```python
from build123d import *

# Parameters (mm, degrees)
BOSS_EXTRUDE1_DEPTH = 30
SKETCH16_W          = 33.4
SKETCH16_H          = 12.9
CUT_EXTRUDE10_DEPTH = 4.5
SKETCH17_W          = 23.45208563
SKETCH17_H          = 12.9
CUT_EXTRUDE11_DEPTH = 192.865838543
CUT_EXTRUDE13_DEPTH = 6.45
SKETCH19_R          = 20
CUT_EXTRUDE14_DEPTH = 8.8
SKETCH21_W          = 33.4
SKETCH21_H          = 12.9
CUT_EXTRUDE15_DEPTH = 191.957455995
SKETCH23_R          = 1.1
CUT_EXTRUDE16_DEPTH = 192.865838543


with BuildPart() as part:
    # Sketch1 → Boss-Extrude1 (new body)
    with BuildSketch(Plane.XY):
        with BuildLine():
            ThreePointArc((187.5, 0), (167.823244805, 26.363741023), (136.951138857, 15))
            Line((136.951138857, 15), (160, 15))
            Line((160, 15), (160, -15))
            Line((160, -15), (136.951138857, -15))
            ThreePointArc((136.951138857, -15), (167.823244805, -26.363741023), (187.5, 0))
        make_face()
        with BuildLine():
            Line((160, 15), (136.951138857, 15))
            ThreePointArc((136.951138857, 15), (132.5, 0), (136.951138857, -15))
            Line((136.951138857, -15), (160, -15))
            Line((160, -15), (160, 15))
        make_face()
        with BuildLine():
            Line((136.951138857, 15), (23.048861143, 15))
            ThreePointArc((23.048861143, 15), (26.363741023, 7.823244805), (27.5, 0))
            ThreePointArc((27.5, 0), (26.363741023, -7.823244805), (23.048861143, -15))
            Line((23.048861143, -15), (136.951138857, -15))
            ThreePointArc((136.951138857, -15), (132.5, 0), (136.951138857, 15))
        make_face()
        with BuildLine():
            ThreePointArc((13.228756555, -15), (-20, 0), (13.228756555, 15))
            Line((13.228756555, 15), (23.048861143, 15))
            ThreePointArc((23.048861143, 15), (-27.5, 0), (23.048861143, -15))
            Line((23.048861143, -15), (13.228756555, -15))
        make_face()
        with BuildLine():
            Line((23.048861143, 15), (13.228756555, 15))
            ThreePointArc((13.228756555, 15), (18.228756555, 8.228756555), (20, 0))
            ThreePointArc((20, 0), (18.228756555, -8.228756555), (13.228756555, -15))
            Line((13.228756555, -15), (23.048861143, -15))
            ThreePointArc((23.048861143, -15), (26.363741023, -7.823244805), (27.5, 0))
            ThreePointArc((27.5, 0), (26.363741023, 7.823244805), (23.048861143, 15))
        make_face()
        with BuildLine():
            Line((0, -15), (0, 15))
            Line((0, 15), (13.228756555, 15))
            ThreePointArc((13.228756555, 15), (-20, 0), (13.228756555, -15))
            Line((13.228756555, -15), (0, -15))
        make_face()
        with BuildLine():
            Line((13.228756555, 15), (0, 15))
            Line((0, 15), (0, -15))
            Line((0, -15), (13.228756555, -15))
            ThreePointArc((13.228756555, -15), (18.228756555, -8.228756555), (20, 0))
            ThreePointArc((20, 0), (18.228756555, 8.228756555), (13.228756555, 15))
        make_face()
    extrude(amount=BOSS_EXTRUDE1_DEPTH)

    # Sketch16 → Cut-Extrude10 (cut)
    with BuildSketch(Plane(origin=(0, 0, 0), x_dir=(-1, 0, 0), z_dir=(0, 0, -1))):
        with Locations((-165.21934279, 0)):
            Rectangle(SKETCH16_W, SKETCH16_H)
    extrude(amount=-CUT_EXTRUDE10_DEPTH, mode=Mode.SUBTRACT)

    # Sketch17 → Cut-Extrude11 (cut, through all)
    with BuildSketch(Plane(origin=(0, 0, 0), x_dir=(-1, 0, 0), z_dir=(0, 0, -1))):
        with Locations((-165.223957185, 0)):
            Rectangle(SKETCH17_W, SKETCH17_H)
    extrude(amount=-CUT_EXTRUDE11_DEPTH, mode=Mode.SUBTRACT)

    # Sketch18 → Cut-Extrude13 (cut, symmetric)
    with BuildSketch(Plane(origin=(0, 0, 0), x_dir=(-1, 0, 0), z_dir=(0, -1, 0))):
        Polygon((-153.49791437, -15), (-153.49791437, -30), (-137.49791437, -30), (-137.49791437, -27.5), align=None)
    extrude(amount=CUT_EXTRUDE13_DEPTH, both=True, mode=Mode.SUBTRACT)

    # Sketch19 → Cut-Extrude14 (cut)
    with BuildSketch(Plane(origin=(0, 0, 0), x_dir=(-1, 0, 0), z_dir=(0, 0, -1))):
        Circle(SKETCH19_R)
    extrude(amount=-CUT_EXTRUDE14_DEPTH, mode=Mode.SUBTRACT)

    # Sketch21 → Cut-Extrude15 (cut, through all)
    with BuildSketch(Plane(origin=(0, 0, 6.5), x_dir=(-1, 0, 0), z_dir=(0, 0, -1))):
        with Locations((-165.21934279, 0)):
            Rectangle(SKETCH21_W, SKETCH21_H)
    extrude(amount=-CUT_EXTRUDE15_DEPTH, mode=Mode.SUBTRACT)

    # Sketch23 → Cut-Extrude16 (cut, through all)
    with BuildSketch(Plane(origin=(0, 0, 0), x_dir=(-1, 0, 0), z_dir=(0, 0, -1))):
        with Locations((-151.71934279, 0)):
            Circle(SKETCH23_R)
        with Locations((-178.71934279, 0)):
            Circle(SKETCH23_R)
    extrude(amount=-CUT_EXTRUDE16_DEPTH, mode=Mode.SUBTRACT)


solid = part.part
```
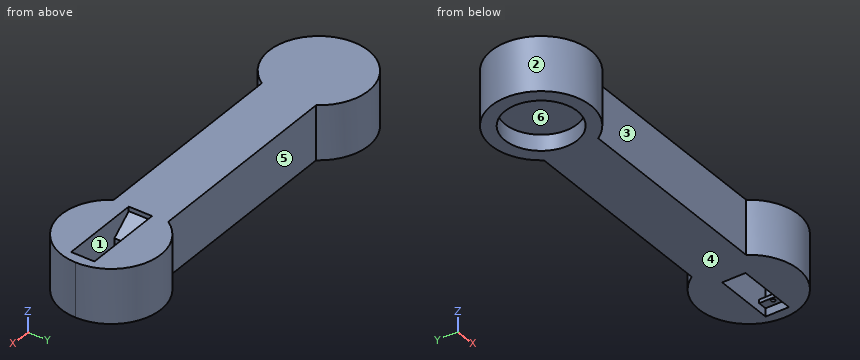
Check sheet for the modelled part. Datum: model origin and axes. Units: mm. Face numbers are marked on the shaded views. A direction names the side the tool comes from. Coordinates: 2 decimals unless noted, no trailing zeros. Write each loop counter-clockwise with the first axis right and the second up, starting at its lowest first coordinate (ties: lowest second). Pieces come first, ordered by that corner, then holes. Notation, with made-up numbers: (55.25, 11.25) -> (75.25, 11.25) arc R30 cw to (75.25, 47.25) -> close; hole circle Ø10 at (-40, 66). An arc over 180 degrees is marked (long way). Use a Markdown table: item, result.
1. Go/stop test with flat-tipped pins: pin 1 Ø5.5 at (x, y) = (178.5, 1) entering from -Z; pin 2 Ø9 at (x, z) = (62.5, 13) entering from +Y; pin 3 Ø5 at (y, z) = (-6.5, 5.5) entering from -X. Record where each tip stops, or that it passes through.
Reported:
| item | result |
|---|---|
| pin 1 | stops at z = 4.5 |
| pin 2 | stops at y = 15 |
| pin 3 | stops at x = -27.21 |
2. Release check for a two-part mould opening along Y. For the marked faces 1, 2 and 3 record: pulls with the +Y half, pulls with the -Y half, needs draft (parallel to the pull), parting line crosses it, or undercut.
Reported:
| item | result |
|---|---|
| face 1 | undercut |
| face 2 | parting line crosses it |
| face 3 | pulls with the -Y half |
3. Sectioned sample at B-B (x = 0). Enter the section's corners in (y, z).
Reported:
| item | result |
|---|---|
| outline | (-27.5, 0) -> (-20, 0) -> (-20, 8.8) -> (20, 8.8) -> (20, 0) -> (27.5, 0) -> (27.5, 30) -> (-27.5, 30) -> close |
4. Scan lines: line 1 along X through (y, z) = (3, 8.5); line 2 along Z through (x, y) = (18, 1.5); line 3 along Y through (x, z) = (108, 10.25). Record each from-to range of solid material in increasing order.
Reported:
| item | result |
|---|---|
| line 1 | x = -27.34 to -19.77, 19.77 to 148.52, 181.92 to 187.34 |
| line 2 | z = 8.8 to 30 |
| line 3 | y = -15 to 15 |
5. Tool access check on the marked faces 4, 5 and 6. Record the directions out of +Z, -Z, +X, -X, +Y, -Y that give a thin tool (end or side, any length) a straight path to the whole face; none if there is none.
Reported:
| item | result |
|---|---|
| face 4 | -Z, +X, -X, +Y, -Y |
| face 5 | +Z, -Z, +Y |
| face 6 | -Z |
6. Sectioned sample at C-C (y = -18). Enter the section's corners in (x, z), plus the area to 3 significant figures.
Reported:
| item | result |
|---|---|
| outline | (-20.79, 0) -> (-8.72, 0) -> (-8.72, 8.8) -> (8.72, 8.8) -> (8.72, 0) -> (20.79, 0) -> (20.79, 30) -> (-20.79, 30) -> close; (139.21, 0) -> (180.79, 0) -> (180.79, 30) -> (139.21, 30) -> close |
| area | 2,340 mm2 |
7. Sectioned sample at A-A (z = 13). Enter the section's corners in (x, y).
Reported:
| item | result |
|---|---|
| outline | (23.05, -15) -> (136.95, -15) arc R27.5 ccw (long way) to (136.95, 15) -> (23.05, 15) arc R27.5 ccw (long way) to start; hole (148.52, -6.45) -> (181.92, -6.45) -> (181.92, 6.45) -> (148.52, 6.45) -> close |
